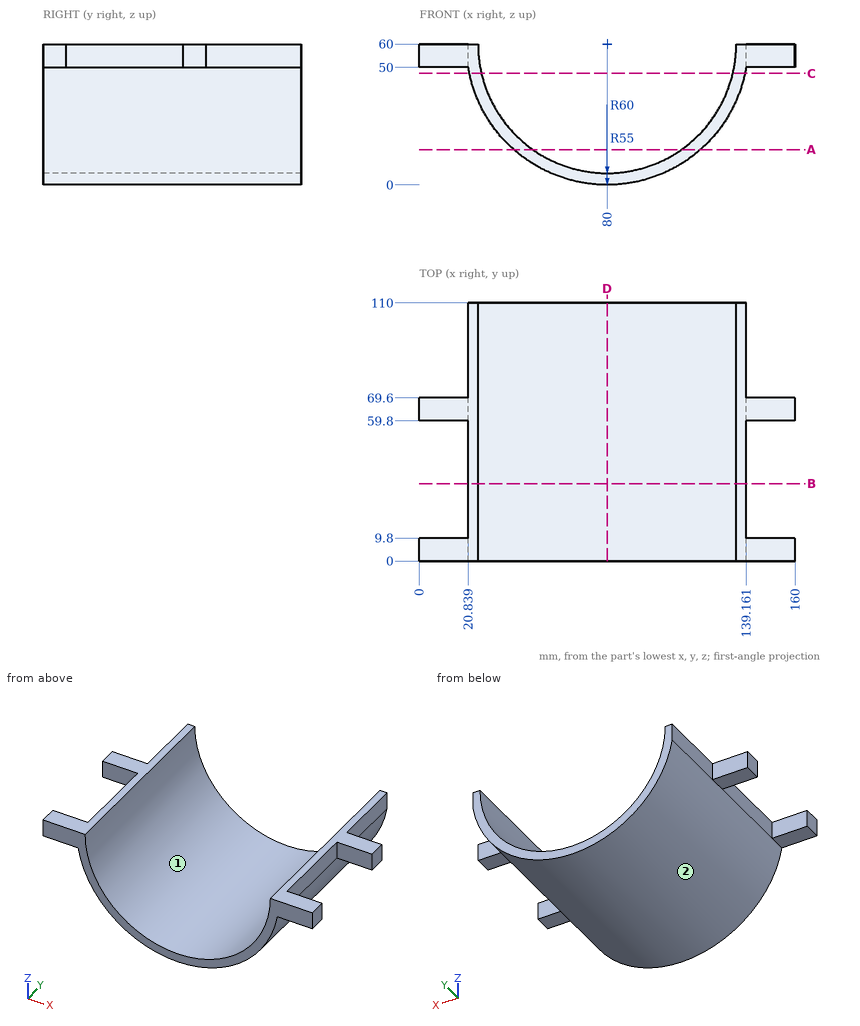
Source: three-view drawing plus pictorial views. Frame: mm from the lowest corner of the part. Coordinates: 2 decimals unless noted, no trailing zeros. Order: outer loops, then holes, each group sorted by start corner. A loop starts at its lowest first (then second) coordinate and runs counter-clockwise, first axis right, second up.
1) Ray query, probe 1 along X at (y, z) = (71.5, 26); probe 2 along X at (y, z) = (37.5, 21.5); probe 3 along Z at (x, y) = (35.5, 80.5) (1 decimal). Return the intervals inside material, ascending.
Result sheet:
probe 1: x = 30.56 to 36.77, 123.23 to 129.44
probe 2: x = 33.98 to 40.72, 119.28 to 126.02
probe 3: z = 19.8 to 27.7
2) Section C-C (z = 47.5). Return loops of the section in (x, y).
Result sheet:
outline: (21.32, 0) - (26.44, 0) - (26.44, 110) - (21.32, 110) - close; (133.56, 0) - (138.68, 0) - (138.68, 110) - (133.56, 110) - close
3) Section D-D (x = 80). Return loops of the section in (y, z), then the cut area to 3 significant figures.
Result sheet:
outline: (0, 0) - (110, 0) - (110, 5) - (0, 5) - close
area: 550 mm2
4) Section B-B (y = 33). Return loops of the section in (x, z), then the cut area to 3 significant figures.
Result sheet:
outline: (20.84, 50) arc R60 ccw to (139.16, 50) - (139.16, 60) - (135, 60) arc R55 cw to (25, 60) - (20.84, 60) - close
area: 892 mm2
5) Section A-A (z = 15). Return loops of the section in (x, y), then the cut area to 3 significant figures.
Result sheet:
outline: (40.31, 0) - (48.38, 0) - (48.38, 110) - (40.31, 110) - close; (111.62, 0) - (119.69, 0) - (119.69, 110) - (111.62, 110) - close
area: 1,770 mm2
6) First-contact query: P1, Ø11, axis at y = 41.5, z = 54, coming from the -X side; P2, Ø3, axis at y = 94, z = 53.5, coming from the +X side; P3, Ø5, axis at y = 93, z = 35, coming from the +X side. Flat tips, straight axial feed; report the tip coordinate or a pass-through.
Result sheet:
P1: stops at x = 20.84
P2: stops at x = 139.16
P3: stops at x = 135.62
7) Draft query along X for the marked faces 1 and 2. Return one class per face: released by +X, released by -X, zero draft, split by the parting line, or undercut.
Result sheet:
face 1: undercut
face 2: split by the parting line
